Model file for the job. Use its own axes, mm. Give positions to 0.01 mm unless a question says otherwise; leave off trailing zeros. Loops run counter-clockwise (first coordinate to the right, second up) from the corner with the lowest first, then second, coordinate; pieces in that order, holes last. Notation, with made-up numbers: (-2.75, 44) - (34.25, 44) arc R15 ccw to (34.25, 67) - close; hole circle Ø4 at (-14.5, 75.25). An arc over 180 degrees is marked (long way). Use a Markdown table: item, result.
from build123d import *

# Parameters (mm, degrees)
F0_W     = 250
F0_H     = 40
F0_R     = 5
F1_DEPTH = 10
F2_R     = 9
F3_DEPTH = 25
F4_R     = 9
F5_DEPTH = 25


with BuildPart() as f1:
    # F0 (on Top) → F1 (new body)
    with BuildSketch(Plane.XY):
        Rectangle(F0_W, F0_H)
        with Locations((-105, 0)):
            Circle(F0_R, mode=Mode.SUBTRACT)
    extrude(amount=F1_DEPTH)

    # F2 (on face) → F3 (cut)
    with BuildSketch(Plane(origin=(0, 0, 0), x_dir=(1, 0, 0), z_dir=(0, 0, -1))):
        with Locations((106, 0)):
            Circle(F2_R)
    extrude(amount=-F3_DEPTH, mode=Mode.SUBTRACT)

    # F4 (on face) → F5 (cut)
    with BuildSketch(Plane(origin=(0, 0, 0), x_dir=(1, 0, 0), z_dir=(0, 0, -1))):
        with Locations((75, 0)):
            Circle(F4_R)
    extrude(amount=-F5_DEPTH, mode=Mode.SUBTRACT)


solid = f1.part
(1) Slice it at D-D, the plane x = -105. Write the cut outline in (y, z), plus the area to 3 significant figures.
Computed:
| item | result |
|---|---|
| outline | (-20, 0) - (-5, 0) - (-5, 10) - (-20, 10) - close; (5, 0) - (20, 0) - (20, 10) - (5, 10) - close |
| area | 300 mm² |
(2) Slice it at B-B, the plane y = 0. Write the cut outline in (x, z).
Computed:
| item | result |
|---|---|
| outline | (-125, 0) - (-110, 0) - (-110, 10) - (-125, 10) - close; (-100, 0) - (66, 0) - (66, 10) - (-100, 10) - close; (84, 0) - (97, 0) - (97, 10) - (84, 10) - close; (115, 0) - (125, 0) - (125, 10) - (115, 10) - close |
(3) Slice it at A-A, the plane x = 106. Write the cut outline in (y, z), plus the area to 3 significant figures.
Computed:
| item | result |
|---|---|
| outline | (-20, 0) - (-9, 0) - (-9, 10) - (-20, 10) - close; (9, 0) - (20, 0) - (20, 10) - (9, 10) - close |
| area | 220 mm² |
(4) Slice it at C-C, the plane z = 8.25. Write the cut outline in (x, y), plus the area to 3 significant figures.
Computed:
| item | result |
|---|---|
| outline | (-125, -20) - (125, -20) - (125, 20) - (-125, 20) - close; hole circle Ø10 at (-105, 0); hole circle Ø18 at (75, 0); hole circle Ø18 at (106, 0) |
| area | 9,410 mm² |
(5) Drill centre lines: probe 1 along X at (y, z) = (-0.5, 1.75); probe 2 along X at (y, z) = (-1.5, 3); probe 3 along X at (y, z) = (-8, 2). Where is each one in solid material? Low to high. Write a range as [from, to].
Computed:
| item | result |
|---|---|
| probe 1 | [-125, -109.97], [-100.03, 66.01], [83.99, 97.01], [114.99, 125] |
| probe 2 | [-125, -109.77], [-100.23, 66.13], [83.87, 97.13], [114.87, 125] |
| probe 3 | [-125, 70.88], [79.12, 101.88], [110.12, 125] |
(6) Pin check, flat tip, straight feed: P1, Ø14.5, axis at x = 75, y = 0, coming from the -Z side. Stop position of the tip, or through.
Computed:
| item | result |
|---|---|
| P1 | through |
(7) Mould opens along X. For faces 1 (the cylindrical face through (114.584, -2.703, 4.93)), 2 (the flat face through (-2, -20, 5)), 3 (the flat face through (125, 0, 5)), 4 (the flat face through (-125, 0, 5)) say: pulls with the +X half, pulls with the -X half, needs draft (parallel to the pull), parting line crosses it, or undercut.
Computed:
| item | result |
|---|---|
| face 1 | undercut |
| face 2 | needs draft |
| face 3 | pulls with the +X half |
| face 4 | pulls with the -X half |
